Source: CAD feature listing. Evaluate the final solid. Frame: model axes, mm. Give positions to 0.01 mm unless a question says otherwise; leave off trailing zeros. Write each loop counter-clockwise with the first axis right and the second up, starting at its lowest first coordinate (ties: lowest second). Pieces come first, ordered by that corner, then holes. Notation, with made-up numbers: M 48,50.25 L 87,50.25 A26 cw 87,80.25 Z; hole C 23,73 d7. An arc over 180 degrees is marked long. Return JSON: item names as keys, results as strings.
```python
from build123d import *

# Parameters (mm, degrees)
BOSS_EXTRUDE4_DEPTH     = 100
SKETCH8_W               = 15
SKETCH8_H               = 2.5
BOSS_EXTRUDE5_DEPTH     = 15
SKETCH9_W               = 15
SKETCH9_H               = 20
BOSS_EXTRUDE6_DEPTH     = 5
CUT_EXTRUDE1_REACH      = 144.354
SKETCH11_R              = 1.5
CUT_EXTRUDE2_DEPTH      = 5
MIRROR4_COPY_1_SKETCH_R = 1.5
MIRROR4_COPY_1_DEPTH    = 5


with BuildPart() as part:
    # Sketch7 → Boss-Extrude4 (new body)
    with BuildSketch(Plane(origin=(0, 0, 0), x_dir=(1, 0, 0), z_dir=(0, 1, 0))):
        Polygon((100, -1), (100, 1), (0, 5), (-100, 1), (-100, -1), (0, -5), align=None)
    extrude(amount=BOSS_EXTRUDE4_DEPTH)

    # Sketch8 → Boss-Extrude5 (add)
    with BuildSketch(Plane.XZ):
        with Locations((-82.5, 0)):
            Rectangle(SKETCH8_W, SKETCH8_H)
    boss_extrude5 = extrude(amount=BOSS_EXTRUDE5_DEPTH)

    # Sketch9 → Boss-Extrude6 (add)
    with BuildSketch(Plane.XZ.offset(15)):
        with Locations((-82.5, 0)):
            Rectangle(SKETCH9_W, SKETCH9_H)
    boss_extrude6 = extrude(amount=BOSS_EXTRUDE6_DEPTH)

    # Mirror1: Boss-Extrude5, Boss-Extrude6 across plane
    add(boss_extrude5.mirror(Plane(origin=(0, 0, 0), x_dir=(0, 0, 1), z_dir=(1, 0, 0))))
    add(boss_extrude6.mirror(Plane(origin=(0, 0, 0), x_dir=(0, 0, 1), z_dir=(1, 0, 0))))

    # Cut-Extrude1: up to this plane
    cut_extrude1_end = Plane(origin=(-100, 100, -1), z_dir=(0.03996803834887159, 0, 0.9992009587217895))
    # Sketch10 → Cut-Extrude1 (cut, up to the surface)
    with BuildSketch(Plane(origin=(-0.199680511, 0, 4.99201278), x_dir=(0.9992009587217895, 0, 0.03996803834887158), z_dir=(-0.039968038348871575, 0, 0.9992009587217894)), mode=Mode.PRIVATE) as cut_extrude1_sk1:
        Polygon((-91.601994525, 67.204299414), (-91.601994525, 93.057612221), (-54.669790851, 93.057612221), align=None)
    cut_extrude1_tool1 = split(extrude(cut_extrude1_sk1.sketch, amount=-CUT_EXTRUDE1_REACH, mode=Mode.PRIVATE), bisect_by=cut_extrude1_end, keep=Keep.BOTH, mode=Mode.PRIVATE)
    # Sketch10 → Cut-Extrude1 (cut, up to the surface)
    with BuildSketch(Plane(origin=(-0.199680511, 0, 4.99201278), x_dir=(0.9992009587217895, 0, 0.03996803834887158), z_dir=(-0.039968038348871575, 0, 0.9992009587217894)), mode=Mode.PRIVATE) as cut_extrude1_sk2:
        Polygon((-91.895790601, 6.886941419), (-54.964445552, 6.635106072), (-91.719500606, 32.739653171), align=None)
    cut_extrude1_tool2 = split(extrude(cut_extrude1_sk2.sketch, amount=-CUT_EXTRUDE1_REACH, mode=Mode.PRIVATE), bisect_by=cut_extrude1_end, keep=Keep.BOTH, mode=Mode.PRIVATE)
    cut_extrude1 = cut_extrude1_tool1.solids().sort_by_distance((-79.427583, 84.439841, 1.822897))[0] + cut_extrude1_tool2.solids().sort_by_distance((-79.662714, 15.420567, 1.813491))[0]
    add(cut_extrude1, mode=Mode.SUBTRACT)

    # Mirror2: Cut-Extrude1 across plane
    add(cut_extrude1.mirror(Plane(origin=(0, 0, 0), x_dir=(0, 0, 1), z_dir=(1, 0, 0))), mode=Mode.SUBTRACT)

    # Sketch11 → Cut-Extrude2 (cut)
    with BuildSketch(Plane(origin=(0, -15, 0), x_dir=(1, 0, 0), z_dir=(0, 1, 0))):
        with Locations(Location((-82.5, 6, 0), (0, 0, 270))):
            Circle(SKETCH11_R)
    cut_extrude2 = extrude(amount=-CUT_EXTRUDE2_DEPTH, mode=Mode.SUBTRACT)

    # Mirror3: Cut-Extrude2 across plane
    add(cut_extrude2.mirror(Plane.XY), mode=Mode.SUBTRACT)

    # Mirror4: Cut-Extrude2 across plane
    add(cut_extrude2.mirror(Plane(origin=(0, 0, 0), x_dir=(0, 0, 1), z_dir=(1, 0, 0))), mode=Mode.SUBTRACT)

    # Mirror4 copy 1 sketch → Mirror4 copy 1 (cut)
    with BuildSketch(Plane(origin=(0, -15, 0), x_dir=(-1, 0, 0), z_dir=(0, 1, 0))):
        with Locations(Location((-82.5, 6, 0), (0, 0, 270))):
            Circle(MIRROR4_COPY_1_SKETCH_R)
    extrude(amount=-MIRROR4_COPY_1_DEPTH, mode=Mode.SUBTRACT)


solid = part.part
```
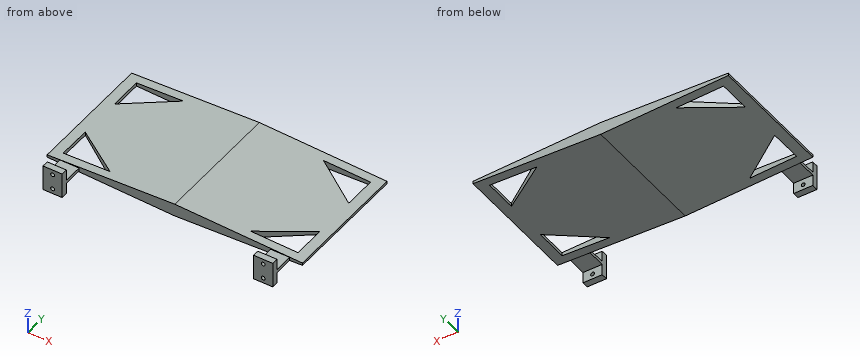
1) Contact query for flat-ended pins moving along their axis: pin 1 Ø5 at (x, y) = (24, 73) entering from -Z; pin 2 Ø3.5 at (x, z) = (82.5, 6) entering from +Y; pin 3 Ø10 at (y, z) = (-14, -5) entering from +X. Output: stop coordinate, or through.
Numbers:
{"pin 1": "stops at z = -4.14", "pin 2": "stops at y = -15", "pin 3": "stops at x = 90"}
2) Cut plane B-B, the plane x = 68. Return the cut outline in (y, z), then the cut area to 3 significant figures.
Numbers:
{"outline": "M 0,-2.28 L 6.72,-2.28 L 6.72,2.28 L 0,2.28 Z; M 15.79,2.28 L 15.92,-2.28 L 83.7,-2.28 L 83.83,2.28 Z; M 93.06,-2.28 L 100,-2.28 L 100,2.28 L 93.06,2.28 Z", "area": "372 mm²"}
3) Cut plane C-C, the plane y = 70.5. Return the cut outline in (x, z).
Numbers:
{"outline": "M -100,-1 L -91.62,-1.34 L -91.73,1.33 L -100,1 Z; M -87.02,1.52 L -86.9,-1.52 L 0,-5 L 86.9,-1.52 L 87.02,1.52 L 0,5 Z; M 91.62,-1.34 L 100,-1 L 100,1 L 91.73,1.33 Z"}
4) Cut plane A-A, the plane y = -3.5. Return the cut outline in (x, z).
Numbers:
{"outline": "M -90,-1.25 L -75,-1.25 L -75,1.25 L -90,1.25 Z; M 75,-1.25 L 90,-1.25 L 90,1.25 L 75,1.25 Z"}
5) Line query: line 1 (X direction, y = -17.75, z = 6); line 2 (Z direction, x = 82.5, y = -18.25); line 3 (Z direction, x = 82, y = -17). Output: solid intervals per line, ascending. Write a range as [from, to].
Numbers:
{"line 1": "x = [-90, -84], [-81, -75], [75, 81], [84, 90]", "line 2": "z = [-10, -7.5], [-4.5, 4.5], [7.5, 10]", "line 3": "z = [-10, -7.41], [-4.59, 4.59], [7.41, 10]"}
6) Cut plane D-D, the plane x = -11.5. Return the cut outline in (y, z), then the cut area to 3 significant figures.
Numbers:
{"outline": "M 0,-4.54 L 100,-4.54 L 100,4.54 L 0,4.54 Z", "area": "908 mm²"}
